The listing builds one solid part. Answer for the finished solid, in the listing's coordinates (mm). Face numbers are marked on the shaded views. A direction names the side the tool comes from. Coordinates: 2 decimals unless noted, no trailing zeros. Order: outer loops, then holes, each group sorted by start corner. A loop starts at its lowest first (then second) coordinate and runs counter-clockwise, first axis right, second up.
```python
from build123d import *

# Parameters (mm, degrees)
SKETCH3_W          = 222.25
SKETCH3_H          = 127
LOWER_DRAWER_DEPTH = 57.15
SKETCH6_W          = 219.71
SKETCH6_H          = 124.46
CUT_EXTRUDE1_DEPTH = 54.61
HANDLE_DEPTH       = 222.25


with BuildPart() as part:
    # Sketch3 → lower drawer (new body)
    with BuildSketch(Plane(origin=(0, 0, 0), x_dir=(1, 0, 0), z_dir=(0, 1, 0))):
        Rectangle(SKETCH3_W, SKETCH3_H)
    extrude(amount=LOWER_DRAWER_DEPTH)

    # Sketch6 → Cut-Extrude1 (cut)
    with BuildSketch(Plane(origin=(0, 57.15, 0), x_dir=(1, 0, 0), z_dir=(0, 1, 0))):
        Rectangle(SKETCH6_W, SKETCH6_H)
    extrude(amount=-CUT_EXTRUDE1_DEPTH, mode=Mode.SUBTRACT)

    # Sketch10 → handle (add)
    with BuildSketch(Plane.ZY.offset(111.125)):
        Polygon((63.5, 57.15), (71.12, 57.15), (71.12, 53.34), (68.58, 53.34), (68.58, 54.61), (63.5, 47.355008126), align=None)
    extrude(amount=-HANDLE_DEPTH)


solid = part.part
```
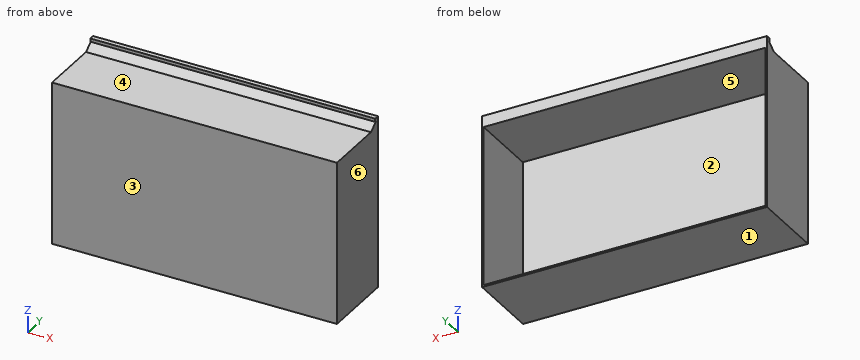
(1) Find section B-B (y = 5.5). Write down the section's boundary in (x, z) (3 decimals).
(2) Consider line 1 (Z direction, x = -15.5, y = 32.5); line 2 (X direction, y = 52, z = -29) (3 decimals); line 3 (Y direction, x = 85, z = -26.5). Determine where each line is inside the solid, lowest interval first.
(3) The mould has two halves that part along Z. Classify the marked faces 1, 2 and 3: released by +Z, released by -Z, zero draft, split by the parting line, or undercut.
(4) Each of these flat-tipped pins is pushed along its axis until it touches: pin 1 Ø3 at (x, y) = (-77.5, 28) entering from +Z; pin 2 Ø5 at (x, z) = (74.5, 32.5) entering from +Y; pin 3 Ø3 at (x, z) = (26, 70) entering from -Y. Where does it stop, or does it pass through?
(5) Find section D-D (y = 50). Write down the section's boundary in (x, z) (3 decimals).
(6) For the marked faces 4, 5 and 6, determine the directions among +Z, -Z, +X, -X, +Y, -Y from which every point of the face is accessible in a straight line to the end or side of a thin tool.
(7) Find section C-C (z = 11). Write down the section's boundary in (x, y) (3 decimals), and give its area (3 significant figures).
(8) Find section A-A (x = 97). Write down the section's boundary in (y, z) (3 decimals), and give its area (3 significant figures).
Findings below:
1. outline: (-111.125, -63.5) - (111.125, -63.5) - (111.125, 63.5) - (-111.125, 63.5) - close; hole (-109.855, -62.23) - (109.855, -62.23) - (109.855, 62.23) - (-109.855, 62.23) - close
2. line 1: z = -63.5 to -62.23, 62.23 to 63.5
2. line 2: x = -111.125 to -109.855, 109.855 to 111.125
2. line 3: y = 0 to 2.54
3. face 1: released by -Z
3. face 2: undercut
3. face 3: zero draft
4. pin 1: stops at z = 63.5
4. pin 2: stops at y = 2.54
4. pin 3: stops at y = 53.34
5. outline: (-111.125, -63.5) - (111.125, -63.5) - (111.125, 65.352) - (-111.125, 65.352) - close; hole (-109.855, -62.23) - (109.855, -62.23) - (109.855, 62.23) - (-109.855, 62.23) - close
6. face 4: +Z, +X, -X, -Y
6. face 5: +Y
6. face 6: +Z, -Z, +X, +Y, -Y
7. outline: (-111.125, 0) - (111.125, 0) - (111.125, 57.15) - (109.855, 57.15) - (109.855, 2.54) - (-109.855, 2.54) - (-109.855, 57.15) - (-111.125, 57.15) - close
7. area: 703 mm2
8. outline: (0, -63.5) - (57.15, -63.5) - (57.15, -62.23) - (2.54, -62.23) - (2.54, 62.23) - (57.15, 62.23) - (57.15, 71.12) - (53.34, 71.12) - (53.34, 68.58) - (54.61, 68.58) - (47.355, 63.5) - (0, 63.5) - close
8. area: 502 mm2
